from build123d import *

# Parameters (mm, degrees)
SKETCH1_W           = 160
SKETCH1_H           = 80
BOSS_EXTRUDE1_DEPTH = 22.5
SKETCH2_W           = 151
SKETCH2_H           = 71
CUT_EXTRUDE1_DEPTH  = 18
SKETCH3_W           = 150
SKETCH3_H           = 70
BOSS_EXTRUDE2_DEPTH = 5
SKETCH4_W           = 18
SKETCH4_H           = 9
CUT_EXTRUDE3_DEPTH  = 13
SKETCH6_R           = 1.6
CUT_EXTRUDE5_DEPTH  = 13
SKETCH5_W           = 25
SKETCH5_H           = 30
CUT_EXTRUDE6_DEPTH  = 13
CHAMFER3_SIZE       = 20


with BuildPart() as part:
    # Sketch1 → Boss-Extrude1 (new body)
    with BuildSketch(Plane(origin=(0, 0, 0), x_dir=(1, 0, 0), z_dir=(0, 1, 0))):
        Rectangle(SKETCH1_W, SKETCH1_H)
    extrude(amount=BOSS_EXTRUDE1_DEPTH)

    # Sketch2 → Cut-Extrude1 (cut)
    with BuildSketch(Plane(origin=(0, 22.5, 0), x_dir=(1, 0, 0), z_dir=(0, 1, 0))):
        Rectangle(SKETCH2_W, SKETCH2_H)
    extrude(amount=-CUT_EXTRUDE1_DEPTH, mode=Mode.SUBTRACT)

    # Sketch3 → Boss-Extrude2 (add)
    with BuildSketch(Plane.ZY.offset(80)):
        with Locations((0, 11.25)):
            Rectangle(SKETCH3_W, SKETCH3_H)
    extrude(amount=BOSS_EXTRUDE2_DEPTH)

    # Sketch4 → Cut-Extrude3 (cut)
    with BuildSketch(Plane(origin=(80, 0, 0), x_dir=(0, 0, -1), z_dir=(1, 0, 0))):
        with Locations((0, 9)):
            Rectangle(SKETCH4_W, SKETCH4_H)
    extrude(amount=-CUT_EXTRUDE3_DEPTH, mode=Mode.SUBTRACT)

    # Sketch6 → Cut-Extrude5 (cut)
    with BuildSketch(Plane(origin=(0, 4.5, 0), x_dir=(1, 0, 0), z_dir=(0, 1, 0))):
        with Locations((57.5, 24.14)):
            Circle(SKETCH6_R)
        with Locations((56.23, -24.12)):
            Circle(SKETCH6_R)
        with Locations((-18.7, -24.14)):
            Circle(SKETCH6_R)
        with Locations((-25.05, 24.12)):
            Circle(SKETCH6_R)
    extrude(amount=-CUT_EXTRUDE5_DEPTH, mode=Mode.SUBTRACT)

    # Sketch5 → Cut-Extrude6 (cut)
    with BuildSketch(Plane.XZ):
        with Locations((57.5, 0)):
            Rectangle(SKETCH5_W, SKETCH5_H)
    extrude(amount=-CUT_EXTRUDE6_DEPTH, mode=Mode.SUBTRACT)

    # Chamfer3
    chamfer3_edges = [part.edges().sort_by_distance(p)[0] for p in [
        (-80, 0, 0),
        (-80, 11.25, 40),
        (-80, 11.25, -40),
    ]]
    chamfer(chamfer3_edges, length=CHAMFER3_SIZE)


solid = part.part
Model file for the job. Use its own axes, mm. A direction names the side the tool comes from. Coordinates: 2 decimals unless noted, no trailing zeros. Order: outer loops, then holes, each group sorted by start corner. A loop starts at its lowest first (then second) coordinate and runs counter-clockwise, first axis right, second up. Notation, with made-up numbers: M -11,-39.75 L -7,-39.75 A22 cw -7,-4.75 Z; hole C 63.5,78 d3. An arc over 180 degrees is marked long. Return JSON: item names as keys, results as strings.
1. Saw through at D-D (x = -71). Give the cut face in (y, z).
Ans:
{"outline": "M -11,-51 L 22.5,-51 L 22.5,-35.5 L 4.5,-35.5 L 4.5,35.5 L 22.5,35.5 L 22.5,51 L -11,51 Z"}
2. Saw through at C-C (y = 30). Give the cut face in (x, z), and give its area (3 significant figures).
Ans:
{"outline": "M -85,-75 L -80,-75 L -80,75 L -85,75 Z", "area": "750 mm^2"}
3. Flat gauge pins, fed straight in: pin 1 (2 mm diameter, centred on x = 77, y = 10.5, fed in from -Z); pin 2 (1.5 mm diameter, centred on x = 41, z = 6.5, fed in from +Y); pin 3 (5 mm diameter, centred on x = -25.05, z = -24.12, fed in from -Y); pin 4 (4 mm diameter, centred on x = -46, y = -2.5, fed in from -Z). Where does each tip first touch, or does it go through?
Ans:
{"pin 1": "z = -40", "pin 2": "y = 4.5", "pin 3": "y = 0", "pin 4": "through"}
4. Tool access for faces 1 (the face through (9, 11, 40)), 2 (the face through (9, 0, -1)), 3 (the face through (45, 2, 0)): list every direction of +Z, -Z, +X, -X, +Y, -Y with a clear straight run to the whole face (end or side of a thin tool).
Ans:
{"face 1": "+Z, +X, +Y, -Y", "face 2": "+Z, -Z, +X, -Y", "face 3": "+Y, -Y"}
5. Saw through at B-B (x = 6.5). Give the cut face in (y, z), and give its area (3 significant figures).
Ans:
{"outline": "M 0,-40 L 22.5,-40 L 22.5,-35.5 L 4.5,-35.5 L 4.5,35.5 L 22.5,35.5 L 22.5,40 L 0,40 Z", "area": "522 mm^2"}
6. Saw through at A-A (z = -4.5). Give the cut face in (x, y).
Ans:
{"outline": "M -85,-23.75 L -80,-23.75 L -80,-20 L -60,0 L 45,0 L 45,4.5 L -75.5,4.5 L -75.5,22.5 L -80,22.5 L -80,46.25 L -85,46.25 Z; M 70,0 L 80,0 L 80,4.5 L 70,4.5 Z; M 75.5,13.5 L 80,13.5 L 80,22.5 L 75.5,22.5 Z"}
7. Drill centre lines: probe 1 along X at (y, z) = (1, -24); probe 2 along X at (y, z) = (2.85, 24.12); probe 3 along Z at (x, y) = (68, 3). Where is each one in solid material? Low to high.
Ans:
{"probe 1": "-85 to -26.65, -23.45 to 55.91, 59.09 to 80", "probe 2": "-85 to -20.3, -17.1 to 54.63, 57.83 to 80", "probe 3": "-40 to -15, 15 to 40"}
8. Pull direction Y, two halves, no side cores. Call faces 4 (the face through (78, 9, -9)), 5 (the face through (-1, 14, 35.5)), 6 (the face through (78, 13.5, 0)), 7 (the face through (-70, -10, 1)): +Y half, -Y half, draft (parallel to the pull), parting line (faces both ways), or undercut.
Ans:
{"face 4": "undercut", "face 5": "draft", "face 6": "undercut", "face 7": "-Y half"}
